The model under review builds one solid part; all positions refer to its coordinate system, in mm. Face numbers are marked on the shaded views. A direction names the side the tool comes from. Coordinates: 2 decimals unless noted, no trailing zeros. Write each loop counter-clockwise with the first axis right and the second up, starting at its lowest first coordinate (ties: lowest second). Pieces come first, ordered by that corner, then holes. Notation, with made-up numbers: (64.5, -18.75) - (110.5, -18.75) arc R14 cw to (110.5, -0.75) - close; hole circle Ø1 at (39, 87). An arc over 180 degrees is marked (long way). Put each result on its own line as item: value.
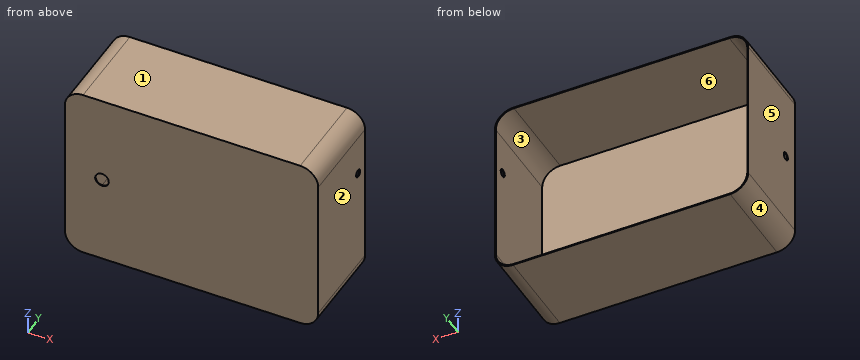
from build123d import *

# Parameters (mm, degrees)
SKETCH1_W                        = 711.2
SKETCH1_H                        = 508
SKETCH1_W_2                      = 706.12
SKETCH1_H_2                      = 502.92
BOSS_EXTRUDE1_DEPTH              = 254
SKETCH2_W                        = 711.2
SKETCH2_H                        = 508
BOSS_EXTRUDE2_DEPTH              = 2.54
FILLET1_R                        = 50.8
SKETCH5_R                        = 19.05
CUT_EXTRUDE1_DEPTH               = 2.54
F_7_8_0_875_DIAMETER_HOLE1_D     = 22.225
F_7_8_0_875_DIAMETER_HOLE1_DEPTH = 2.54
F_7_8_0_875_DIAMETER_HOLE2_D     = 22.225
F_7_8_0_875_DIAMETER_HOLE2_DEPTH = 2.54


with BuildPart() as part:
    # Sketch1 → Boss-Extrude1 (new body)
    with BuildSketch(Plane(origin=(0, 0, 0), x_dir=(1, 0, 0), z_dir=(0, 1, 0))):
        Rectangle(SKETCH1_W, SKETCH1_H)
        Rectangle(SKETCH1_W_2, SKETCH1_H_2, mode=Mode.SUBTRACT)
    extrude(amount=BOSS_EXTRUDE1_DEPTH)

    # Sketch2 → Boss-Extrude2 (add)
    with BuildSketch(Plane.XZ):
        Rectangle(SKETCH2_W, SKETCH2_H)
    extrude(amount=BOSS_EXTRUDE2_DEPTH)

    # Fillet1
    fillet1_edges = [part.edges().sort_by_distance(p)[0] for p in [
        (353.06, 127, 251.46),
        (353.06, 127, -251.46),
        (-353.06, 127, -251.46),
        (-353.06, 127, 251.46),
        (355.6, 125.73, 254),
        (-355.6, 125.73, 254),
        (-355.6, 125.73, -254),
        (355.6, 125.73, -254),
    ]]
    fillet(fillet1_edges, radius=FILLET1_R)

    # Sketch5 → Cut-Extrude1 (cut)
    with BuildSketch(Plane(origin=(0, 0, 0), x_dir=(1, 0, 0), z_dir=(0, 1, 0))):
        with Locations((-251.46, 0)):
            Circle(SKETCH5_R)
    extrude(amount=-CUT_EXTRUDE1_DEPTH, mode=Mode.SUBTRACT)

    # 7/8 (0.875) Diameter Hole1
    with Locations(Plane.ZY.offset(355.6)):
        with Locations((0, 48.26)):
            Hole(F_7_8_0_875_DIAMETER_HOLE1_D / 2, depth=F_7_8_0_875_DIAMETER_HOLE1_DEPTH)

    # 7/8 (0.875) Diameter Hole2
    with Locations(Plane(origin=(355.6, 0, 0), x_dir=(0, 0, -1), z_dir=(1, 0, 0))):
        with Locations((-88.9, 215.9)):
            Hole(F_7_8_0_875_DIAMETER_HOLE2_D / 2, depth=F_7_8_0_875_DIAMETER_HOLE2_DEPTH)


solid = part.part
1. Consider section C-C on y = 110.5. State the section outline as (x, z) points.
Determined:
outline: (-355.6, -203.2) arc R50.8 ccw to (-304.8, -254) - (304.8, -254) arc R50.8 ccw to (355.6, -203.2) - (355.6, 203.2) arc R50.8 ccw to (304.8, 254) - (-304.8, 254) arc R50.8 ccw to (-355.6, 203.2) - close; hole (-353.06, -200.66) arc R50.8 ccw to (-302.26, -251.46) - (302.26, -251.46) arc R50.8 ccw to (353.06, -200.66) - (353.06, 200.66) arc R50.8 ccw to (302.26, 251.46) - (-302.26, 251.46) arc R50.8 ccw to (-353.06, 200.66) - close
2. Consider section D-D on z = 88.9. State the section outline as (x, y) points, plus the area to 3 significant figures.
Determined:
outline: (-355.6, -2.54) - (355.6, -2.54) - (355.6, 204.79) - (353.06, 204.79) - (353.06, 0) - (-353.06, 0) - (-353.06, 254) - (-355.6, 254) - close; (353.06, 227.01) - (355.6, 227.01) - (355.6, 254) - (353.06, 254) - close
area: 3,040 mm^2
3. For pin 1 Ø2 at (x, z) = (-74.5, -81) entering from +Y, flat-tipped, find the tip position at first contact; note if it passes through.
Determined:
pin 1: stops at y = 0
4. Machinability: for the marked faces 5 and 6, which of the approach directions +Z, -Z, +X, -X, +Y, -Y give a long, thin tool a straight path to every point of the face, cutting with its end or side? Answer none if there is none.
Determined:
face 5: +Z, -Z, -X, +Y, -Y
face 6: +Y
5. Consider section B-B on x = -251.46. State the section outline as (y, z) points.
Determined:
outline: (-2.54, -254) - (254, -254) - (254, -251.46) - (0, -251.46) - (0, -19.05) - (-2.54, -19.05) - close; (-2.54, 19.05) - (0, 19.05) - (0, 251.46) - (254, 251.46) - (254, 254) - (-2.54, 254) - close
6. To check wall thickness, follow probe 1 along Z at (x, y) = (-251.46, -0.45); probe 2 along Z at (x, y) = (254, 178); probe 3 along X at (y, z) = (165, 89). State the ranges of each line that lie inside material, in increasing order.
Determined:
probe 1: z = -254 to -19.05, 19.05 to 254
probe 2: z = -254 to -251.46, 251.46 to 254
probe 3: x = -355.6 to -353.06, 353.06 to 355.6
7. The part is to be moulded in two halves that separate along Z. For the marked faces 1, 2, 3 and 4, say which applies: +Z half, -Z half, draft (parallel to the pull), parting line (faces both ways), or undercut.
Determined:
face 1: +Z half
face 2: draft
face 3: undercut
face 4: -Z half
8. Consider section A-A on z = 0. State the section outline as (x, y) points.
Determined:
outline: (-355.6, -2.54) - (-270.51, -2.54) - (-270.51, 0) - (-353.06, 0) - (-353.06, 37.15) - (-355.6, 37.15) - close; (-355.6, 59.37) - (-353.06, 59.37) - (-353.06, 254) - (-355.6, 254) - close; (-232.41, -2.54) - (355.6, -2.54) - (355.6, 254) - (353.06, 254) - (353.06, 0) - (-232.41, 0) - close
